Here's the drawing with two shaded views (mm, measured from the low corner). I have some questions. A direction names the side the tool comes from. Round coordinates to 2 decimals unless told otherwise and drop trailing zeros. Order: outer loops, then holes, each group sorted by start corner. A loop starts at its lowest first (then second) coordinate and runs counter-clockwise, first axis right, second up. Notation, with made-up numbers: (-37, -27) -> (-2, -27) arc R8 ccw to (-2, -19) -> close; hole circle Ø2 at (14.25, 5). An arc over 180 degrees is marked (long way). Use a Markdown table: item, result. Add a question column.
Q1. I'm going to push flat-ended pins straight in: pin 1 Ø2 at (x, z) = (7, 4) entering from -Y; pin 2 Ø0.6 at (x, y) = (4, 6) entering from +Z; pin 3 Ø1.4 at (x, z) = (8.5, 3.5) entering from -Y. Where does each tip first touch, or does it pass through?
Q2. If we section it at A-A on y = 2.75: List the corners of the cut face in (x, z) for me, plus the area to 3 significant figures.
Q3. I need wall thicknesses on line 1 along Y through (x, z) = (4.5, 8.25); line 2 along Y through (x, z) = (4.5, 7.55); line 3 along Z through (x, y) = (5.25, 6). Which ranges of each line are inside material? Lowest first, please. Write a range as [from, to].
Q4. We'd pull the mould along Y, two halves only. Please class the marked faces 4, 5 and 6: +Y half, -Y half, draft (parallel to the pull), parting line (faces both ways), or undercut.
Q5. If we section it at C-C on y = 1: List the corners of the cut face in (x, z) for me.
Q6. For the marked faces 1, 2 and 3, which set-ups out of +Z, -Z, +X, -X, +Y, -Y let a thin tool reach every point of the face, with its end or its side?
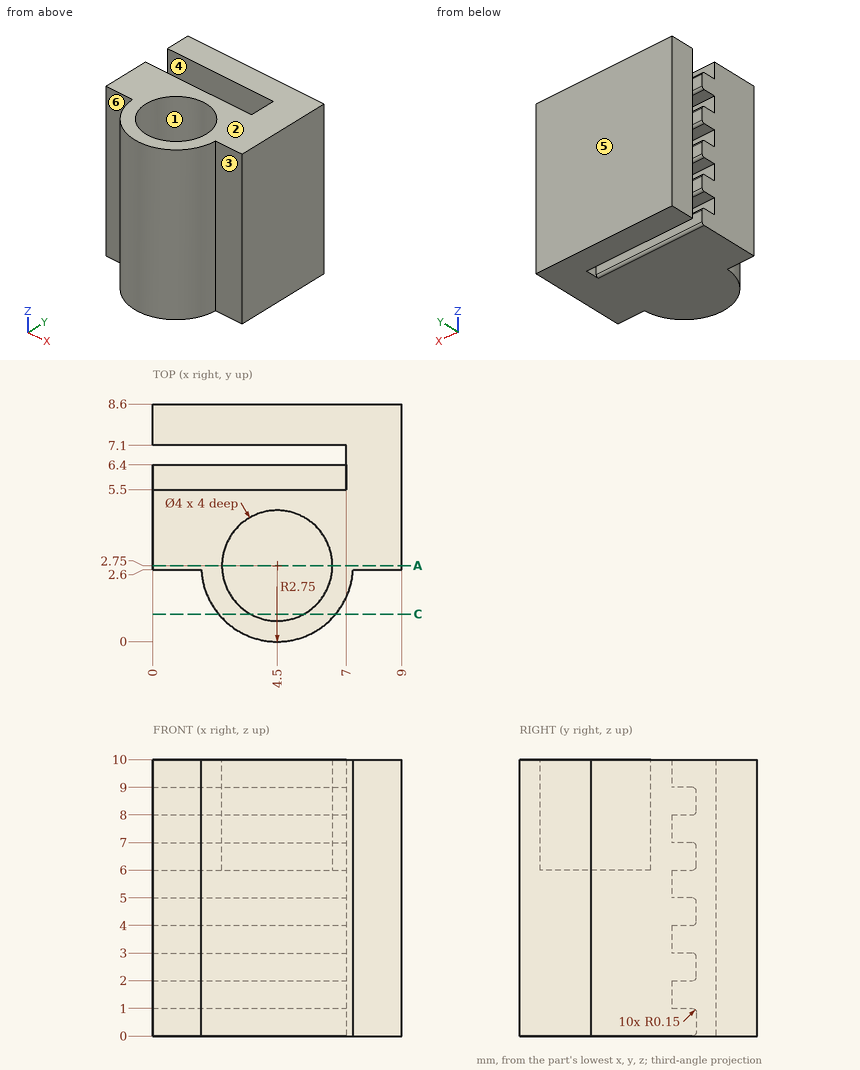
Answer below:
| question | item | result |
|---|---|---|
| 1 | pin 1 | y = 0.45 |
| 1 | pin 2 | z = 9 |
| 1 | pin 3 | y = 2.6 |
| 2 | outline | (0, 0) -> (9, 0) -> (9, 10) -> (6.5, 10) -> (6.5, 6) -> (2.5, 6) -> (2.5, 10) -> (0, 10) -> close |
| 2 | area | 74.0 mm² |
| 3 | line 1 | [0, 0.75], [4.75, 6.4], [7.1, 8.6] |
| 3 | line 2 | [0, 0.75], [4.75, 5.5], [7.1, 8.6] |
| 3 | line 3 | [0, 1], [2, 3], [4, 5], [6, 7], [8, 9] |
| 4 | face 4 | undercut |
| 4 | face 5 | +Y half |
| 4 | face 6 | -Y half |
| 5 | outline | (2.38, 0) -> (6.62, 0) -> (6.62, 10) -> (5.47, 10) -> (5.47, 6) -> (3.53, 6) -> (3.53, 10) -> (2.38, 10) -> close |
| 6 | face 1 | +Z |
| 6 | face 2 | +Z, +X, -X, +Y, -Y |
| 6 | face 3 | +Z, -Z, +X, -Y |
